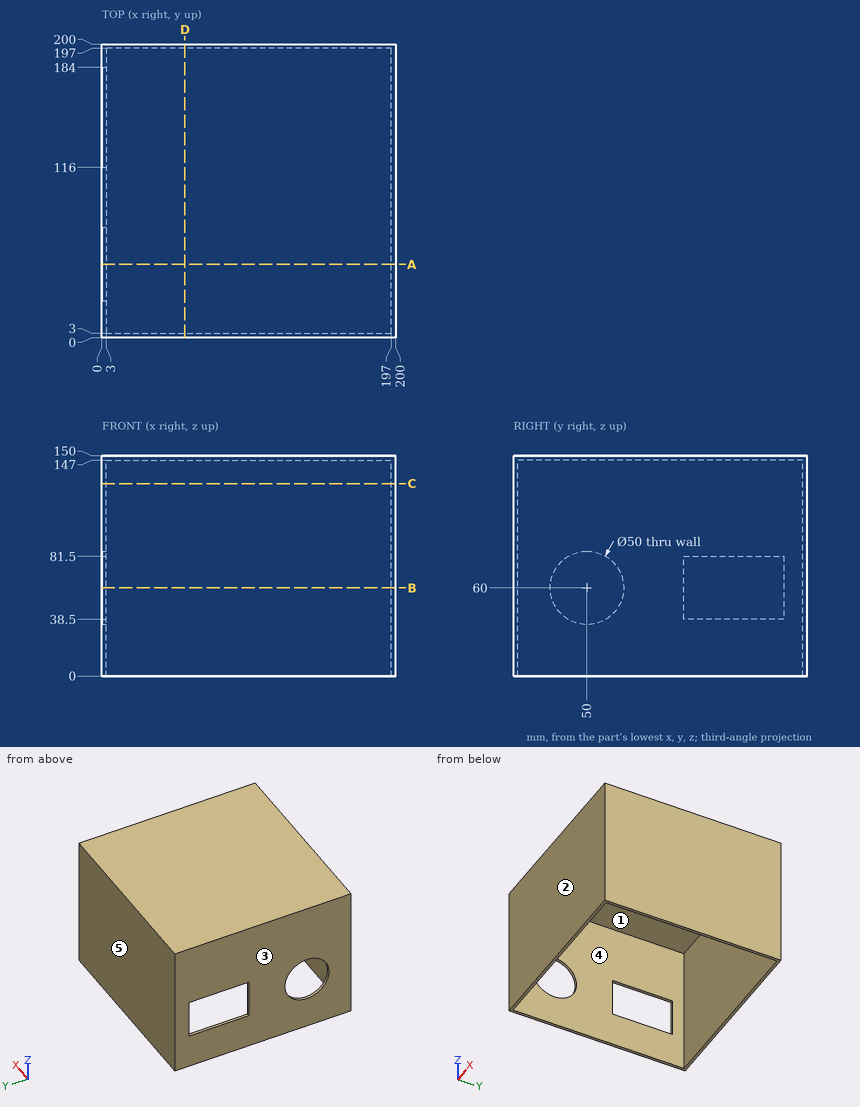
Could you check a few things on this drawing? It's one solid part, dimensions in mm from its lowest x, y, z. A direction names the side the tool comes from. Give positions to 0.01 mm unless a question says otherwise; leave off trailing zeros. Order: outer loops, then holes, each group sorted by start corner. A loop starts at its lowest first (then second) coordinate and runs counter-clockwise, first axis right, second up. Notation, with made-up numbers: (53, 79.25) -> (84, 79.25) arc R8 cw to (84, 91.25) -> close; hole circle Ø1 at (-7.5, -20). An arc over 180 degrees is marked (long way). Use CSV: the item, a comma, the result in double quotes. Start each with the question number.
Item 1: I'm going to push flat-ended pins straight in: P1, Ø6, axis at x = 174.5, z = 76, coming from the -Y side; P2, Ø1.5, axis at x = 73, y = 90.5, coming from the -Z side. Where does each tip first touch, or does it pass through?
Item 2: Suppose I cut it at B-B (z = 60). List the corners of the cut face in (x, y) for me, and give its area (3 significant figures).
Item 3: On a 3-axis mill with a long thin cutter (end or side, diameter ignored), from which of +Z, -Z, +X, -X, +Y, -Y can I reach the whole of each face in a straight line? I mean the marked faces 4 and 5. Say none if no direction works.
Item 4: Suppose I cut it at A-A (y = 50). List the corners of the cut face in (x, z) for me, and give its area (3 significant figures).
Item 5: Thinking about a two-plate mould opening in X: for the marked faces 1, 2 and 3, which applies, pulls with the +X half, pulls with the -X half, needs draft (parallel to the pull), parting line crosses it, or undercut?
Item 6: Suppose I cut it at C-C (z = 131). List the corners of the cut face in (x, y) for me, and give its area (3 significant figures).
Item 7: If I drill on probe 1 along Y at (x, z) = (2.25, 60); probe 2 along X at (y, z) = (160, 111.5), over which ranges is the centre line in solid material (lowest first)? Write a range as [from, to].
Item 8: Suppose I cut it at D-D (x = 56.5). List the corners of the cut face in (y, z) for me, and give its area (3 significant figures).
Answer block:
1,P1,"stops at y = 0"
1,P2,"stops at z = 147"
2,outline,"(0, 0) -> (200, 0) -> (200, 200) -> (0, 200) -> (0, 184) -> (3, 184) -> (3, 197) -> (197, 197) -> (197, 3) -> (3, 3) -> (3, 25) -> (0, 25) -> close; (0, 75) -> (3, 75) -> (3, 116) -> (0, 116) -> close"
2,area,"2,010 mm^2"
3,face 4,"-Z"
3,face 5,"+Z, -Z, +X, -X, +Y"
4,outline,"(0, 0) -> (3, 0) -> (3, 35) -> (0, 35) -> close; (0, 85) -> (3, 85) -> (3, 147) -> (197, 147) -> (197, 0) -> (200, 0) -> (200, 150) -> (0, 150) -> close"
4,area,"1,330 mm^2"
5,face 1,"undercut"
5,face 2,"needs draft"
5,face 3,"pulls with the -X half"
6,outline,"(0, 0) -> (200, 0) -> (200, 200) -> (0, 200) -> close; hole (3, 3) -> (197, 3) -> (197, 197) -> (3, 197) -> close"
6,area,"2,360 mm^2"
7,probe 1,"y = [0, 25], [75, 116], [184, 200]"
7,probe 2,"x = [0, 3], [197, 200]"
8,outline,"(0, 0) -> (3, 0) -> (3, 147) -> (197, 147) -> (197, 0) -> (200, 0) -> (200, 150) -> (0, 150) -> close"
8,area,"1,480 mm^2"
